Read the model definition and answer for the solid it produces. Units are mm, in the model's axes. A direction names the side the tool comes from. Give positions to 0.01 mm unless a question says otherwise; leave off trailing zeros. Loops run counter-clockwise (first coordinate to the right, second up) from the corner with the lowest first, then second, coordinate; pieces in that order, holes last. Notation, with made-up numbers: (57, -27.5) - (88, -27.5) arc R6 cw to (88, -18.5) - close; hole circle Ø11 at (-9, 85.5). An arc over 180 degrees is marked (long way). Write item = value, one per line.
Autodesk Inventor part; units mm, degrees
ref_plane "Work Plane1" through (1.525, 0, 0) normal (0, 0, 1) x (1, 0, 0)
ref_plane "YZ Plane" through (0, 0, 0) normal (1, 0, 0) x (0, 1, 0)
ref_plane "XZ Plane" through (0, 0, 0) normal (0, 1, 0) x (-1, 0, 0)
sketch "Szkic1" plane through (0, 0, 0) normal (0, 0, 1) x (1, 0, 0)
  line L0 (0, 3) -> (60, 3)
  line L1 (60, 3) -> (60, 0)
  line L2 (60, 0) -> (0, 0)
  line L3 (-12, 0) -> (72, 0)
  line L4 (0, -0.6) -> (0, 3.6)
  line L5 (0, 3) -> (0, 0)
  dimension "d2" = 6
  dimension "d59" = 60
revolve "Bryła" add sketch "Szkic1" angle 360 about axis through (60, 0, 0) along (-1, 0, 0)
sketch "Szkic2" plane through (0, 0, 0) normal (-1, 0, 0) x (0, 0, 1)
  line L0 (0, 5.7735) -> (5, 2.8868)
  line L1 (5, 2.8868) -> (5, -2.8868)
  line L2 (5, -2.8868) -> (0, -5.7735)
  line L3 (0, -5.7735) -> (-5, -2.8868)
  line L4 (-5, -2.8868) -> (-5, 2.8868)
  line L5 (-5, 2.8868) -> (0, 5.7735)
  line L6 (-7, 0) -> (7, 0)
  line L7 (0, 8.0829) -> (0, -8.0829)
  point P0 (0, 0)
  point P1 (0, 0)
  dimension "d11" = 10
extrude "Głowica" add sketch "Szkic2" along normal blind 4.38
sketch "Szkic4" plane through (0, 0, 0) normal (0, 0, 1) x (1, 0, 0)
  line L0 (-3.8026, 6) -> (-4.38, 5)
  line L1 (-1.1, 0) -> (-0.234, 0)
  line L2 (-5.2092, 0) -> (0.5952, 0)
  line L3 (-4.38, 6) -> (-3.8026, 6)
  line L4 (-4.38, 5) -> (-4.38, 6)
  line L5 (0, 7.2) -> (0, -1.2)
  dimension "d65" = 10
  dimension "d67" = 30
  dimension "d68" = 12
  dimension "d69" = 4.38
revolve "Faza1" cut sketch "Szkic4" angle 360 about axis through (-1.1, 0, 0) along (1, 0, 0)
thread "Gwint"
chamfer "Faza2" distance 0.6135 distance2 0.6136 1 edges at (60, -3, 0) measured on face at (60, 0.0929, 0.8807)
fillet "Fillet" radius 0.3 1 edges at (0, -3, 0)
ref_plane "Work Plane1" through (1.525, 0, 0) normal (0, 0, 1) x (1, 0, 0)
equation "\"d71\" = RR1"
equation "\"d11\" = SW"
equation "\"d3\" = KOH"
equation "\"d15\" = GEL"
equation "\"d6\" = -0.5 * SPD + 0.5 * GD"
equation "\"d2\" = GD"
equation "\"d59\" = NLG"
equation "\"d65\" = SW"
equation "\"d67\" = ANG1"
equation "\"d68\" = 1.2 * SW"
equation "\"d69\" = KOH"
equation "\"NLG\" = 60"
equation "\"GD\" = NND"
equation "\"BDM\" = NND"
equation "\"KOH\" = 4.38"
equation "\"GEL\" = 18"
equation "\"SW\" = 10"
equation "\"SPD\" = NND - 1.2269 * PTC"
equation "\"SD2\" = NND"
equation "\"SD\" = 0"
equation "\"ANG1\" = 30deg"
equation "\"GAL\" = 0.61345 * PTC"
equation "\"GUL\" = 0.61345 * PTC"
equation "\"RR\" = 0.1"
equation "\"RR1\" = 0.3"
equation "\"GD1\" = THREADDIA - 1.2269 * PTC"
equation "\"THREADDIA\" = 6"
equation "\"TOA\" = 30deg"
equation "\"PTC\" = 1"
equation "\"KOH1\" = 2.8"
equation "\"NND\" = 6"
equation "\"E0\" = 1.155 * SW"
properties part number "ANSI B18.2.3.5M - M6 x 1 x 60" material "Stal, miękka"
1) Find the intervals of material crossed by probe 1 along X at (y, z) = (-2, -4.5); probe 2 along Y at (x, z) = (43, 0); probe 3 along X at (y, z) = (-3.25, 4), in increasing order.
Output:
probe_1 = -4.38 to 0
probe_2 = -3 to 3
probe_3 = -4.29 to 0
2) A tool of negligible diameter and unlimited length cuts with its end or side. For faces 1 (the face through (0, -1.2, -3.4)), 2 (the face through (-2, 0, 5)), from which of +Z, -Z, +X, -X, +Y, -Y can it reach the whole face along a straight path? Write none if from no direction.
Output:
face_1 = +X
face_2 = +Z, +X, -X, +Y, -Y
3) A cutting plane is placed at A-A on x = 40. Determine the outline of the cut face in (y, z), then the cut area to 3 significant figures.
Output:
outline = circle Ø6 at (0, 0)
area = 28.3 mm²
4) Each of these flat-tipped pins is pushed along its axis until it touches: P1, Ø1.5, axis at x = 42, z = -3, coming from the -Y side; P2, Ø1.5, axis at x = 52.5, z = -0.5, coming from the -Y side; P3, Ø5, axis at x = 19, y = 1, coming from the +Z side. Where does it stop, or does it pass through?
Output:
P1 = -1.98
P2 = -3
P3 = 3
